Autodesk Inventor part; units mm, degrees
ref_plane "YZ Plane" through (0, 0, 0) normal (1, 0, 0) x (0, 1, 0)
ref_plane "XZ Plane" through (0, 0, 0) normal (0, 1, 0) x (-1, 0, 0)
ref_plane "XY Plane" through (0, 0, 0) normal (0, 0, 1) x (1, 0, 0)
sketch "草图1" plane through (0, 0, 0) normal (0, 1, 0) x (-1, 0, 0)
  circle A0 centre (0, 0) radius 55
  dimension "d0" = 110
extrude "拉伸1" add sketch "草图1" along normal blind 100
sketch "草图2" plane through (0, 100, 0) normal (0, 1, 0) x (1, 0, 0)
  circle A0 centre (0, 0) radius 35
  dimension "d3" = 70
extrude "拉伸2" cut sketch "草图2" against normal blind 100
sketch "草图3" plane through (0, 100, 0) normal (0, 1, 0) x (1, 0, 0)
  circle A0 centre (0, 0) radius 45
  circle A1 centre (0, 0) radius 55
  dimension "d6" = 90
  dimension "d7" = 110
extrude "拉伸3" cut sketch "草图3" against normal blind 40
thread "螺纹1"
chamfer "倒角1" distance 10 angle 45 1 edges at (55, 0, 0)
chamfer "倒角2" distance 5 angle 45 1 edges at (-45, 100, 0)
fillet "圆角1" radius 3 1 edges at (-45, 60, 0)
properties part number "液压杆盖" material "不锈钢"
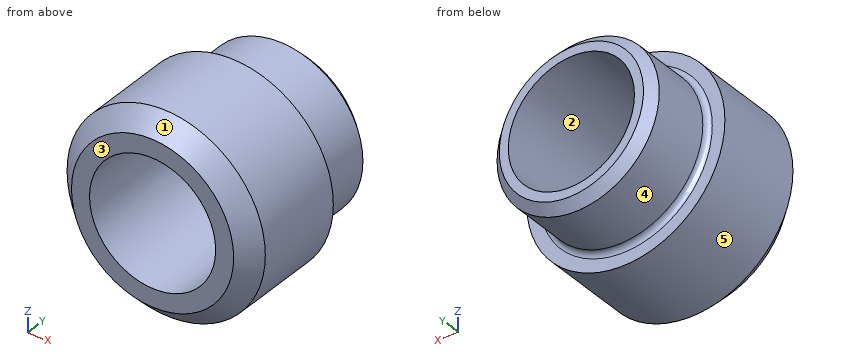
Part model, mm, in its own coordinate system. Face numbers are marked on the shaded views. A direction names the side the tool comes from. Give positions to 0.01 mm unless a question says otherwise; leave off trailing zeros. Order: outer loops, then holes, each group sorted by start corner. A loop starts at its lowest first (then second) coordinate and runs counter-clockwise, first axis right, second up. Notation, with made-up numbers: M 55.25,-6 L 62.25,-6 A31 ccw 62.25,32 Z; hole C 83,39.25 d10. An arc over 180 degrees is marked long. Use a Markdown table: item, result. Add a question column.
(1) Saw through at D-D, the plane y = 40. Give the cut face in (x, z), and give its area (3 significant figures).
(2) Saw through at C-C, the plane y = 85.5. Give the cut face in (x, z), and give its area (3 significant figures).
(3) Drop flat-ended pins along their axis: P1, Ø2, axis at y = 86.5, z = -35.5, coming from the -X side; P2, Ø10, axis at y = 66, z = -1, coming from the -X side; P3, Ø1.5, axis at y = 65, z = 10.5, coming from the -X side. Give the stop position or say it passes through.
(4) Saw through at B-B, the plane x = 0. Give the cut face in (y, z).
(5) Probe line 1 along X through (y, z) = (68, 0); line 2 along X through (y, z) = (45, 0). List the from-to ranges inside material, lowest first. Write a range as [from, to].
(6) Mould opens along X. For the marked faces 1, 2 and 3 say: +X half, -X half, draft (parallel to the pull), parting line (faces both ways), or undercut.
(7) 3-axis set-ups, long thin cutter, end or side, ignore diameter. For the marked faces 4 and 5: which of +Z, -Z, +X, -X, +Y, -Y reach the whole face in a straight line?
(8) Saw through at A-A, the plane z = 0. Give the cut face in (x, y).
Answer key:
| question | item | result |
|---|---|---|
| 1 | outline | C 0,0 d110; hole C 0,0 d70 |
| 1 | area | 5,650 mm^2 |
| 2 | outline | C 0,0 d90; hole C 0,0 d70 |
| 2 | area | 2,510 mm^2 |
| 3 | P1 | x = -28.89 |
| 3 | P2 | x = -45.75 |
| 3 | P3 | x = -43.93 |
| 4 | outline | M 0,-45 L 10,-55 L 60,-55 L 60,-48 A3 cw 63,-45 L 95,-45 L 100,-40 L 100,-35 L 0,-35 Z; M 0,35 L 100,35 L 100,40 L 95,45 L 63,45 A3 cw 60,48 L 60,55 L 10,55 L 0,45 Z |
| 5 | line 1 | [-45, -35], [35, 45] |
| 5 | line 2 | [-55, -35], [35, 55] |
| 6 | face 1 | parting line |
| 6 | face 2 | undercut |
| 6 | face 3 | draft |
| 7 | face 4 | +Y |
| 7 | face 5 | +Y, -Y |
| 8 | outline | M -55,10 L -45,0 L -35,0 L -35,100 L -40,100 L -45,95 L -45,63 A3 cw -48,60 L -55,60 Z; M 35,0 L 45,0 L 55,10 L 55,60 L 48,60 A3 cw 45,63 L 45,95 L 40,100 L 35,100 Z |
